Could you check a few things on this model? Use its own coordinates, in mm. Face numbers are marked on the shaded views. A direction names the side the tool comes from. Round coordinates to 2 decimals unless told otherwise and drop trailing zeros. Write each loop counter-clockwise with the first axis right and the second up, starting at its lowest first coordinate (ties: lowest second). Pieces come first, ordered by that corner, then holes. Notation, with made-up numbers: (36, 37) -> (92, 37) arc R15 cw to (92, 66) -> close; hole circle Ø5 at (49.5, 23). An arc over 180 degrees is marked (long way). Return JSON: item names as keys, results as strings.
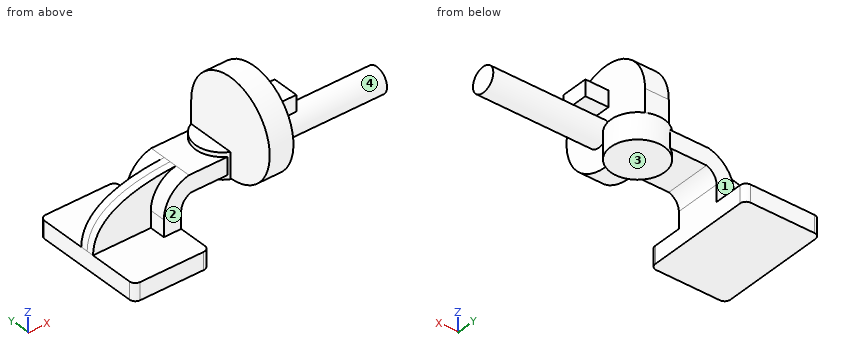
from build123d import *

# Parameters (mm, degrees)
F1_DEPTH  = 63.5
F0_W      = 21.3422756978
F0_H      = 19.05
F2_DEPTH  = 25.4
F3_DEPTH  = 7.9375
F5_R      = 6.35
F6_W      = 26.030293598
F6_H      = 52.8502463959
F7_DEPTH  = 25.4
F7_FACE_W = 26.030293598
F7_FACE_H = 52.8502463959
F9_W      = 29.2156040668
F9_H      = 17.6097750664
F10_DEPTH = 25.4
F12_R     = 13.6846052914
F13_DEPTH = 127


with BuildPart() as f1:
    # F0 (on Front) → F1 (new body, symmetric)
    with BuildSketch(Plane.XZ):
        Polygon((41.275, -9.525), (41.275, 9.525), (22.225, 9.525), (-41.275, 9.525), (-41.275, -9.525), align=None)
    extrude(amount=F1_DEPTH, both=True)

    # F0 (on Front) → F2 (join, symmetric)
    with BuildSketch(Plane.XZ):
        with BuildLine():
            Line((22.225, 9.525), (41.275, 9.525))
            Line((41.275, 9.525), (41.275, 27.7654680662))
            ThreePointArc((41.275, 27.7654680662), (44.31804227, 37.1119372292), (52.28054152, 42.8752))
            Line((52.28054152, 42.8752), (85.9294086695, 42.8752))
            Line((85.9294086695, 42.8752), (85.9294086695, 61.9252))
            Line((85.9294086695, 61.9252), (49.8789382336, 61.9252))
            ThreePointArc((49.8789382336, 61.9252), (30.0050422989, 49.7406107598), (22.225, 27.7654680662))
            Line((22.225, 27.7654680662), (22.225, 9.525))
        make_face()
        with Locations((96.6005465184, 52.4002)):
            Rectangle(F0_W, F0_H)
    extrude(amount=F2_DEPTH, both=True)

    # F0 (on Front) → F3 (join, symmetric)
    with BuildSketch(Plane.XZ):
        with BuildLine():
            Line((-41.275, 9.525), (22.225, 9.525))
            Line((22.225, 9.525), (22.225, 27.7654680662))
            ThreePointArc((22.225, 27.7654680662), (30.0050422989, 49.7406107598), (49.8789382336, 61.9252))
            add(Edge.make_bspline(
                [(-41.275, 9.525), (-40.6103878044, 51.4096161185), (12.72025149, 60.2582759139), (49.8789382336, 61.9252)],
                knots=[0, 0, 0, 0, 105.1419108421, 105.1419108421, 105.1419108421, 105.1419108421], degree=3))
        make_face()
    extrude(amount=F3_DEPTH, both=True)

    # F0 (on Front) → F4 (revolve)
    with BuildSketch(Plane.XZ):
        Polygon((107.2716843673, 61.9252), (107.2716843673, 42.8752), (107.2716843673, 38.1), (136.7294086695, 38.1), (136.7294086695, 66.675), (107.2716843673, 66.675), align=None)
    revolve(axis=Axis((107.2716843673, 0, 52.3875), (0, 0, -1)))

    # F5
    f5_edges = [f1.edges().sort_by_distance(p)[0] for p in [
        (41.275, -63.5, 0),
        (41.275, 63.5, 0),
        (-41.275, 63.5, 0),
        (-41.275, -63.5, 0),
    ]]
    fillet(f5_edges, radius=F5_R)

    # F6 (on face) → F7 (join)
    with BuildSketch(Plane.XY.offset(66.675)):
        with Locations((107.5195462284, -0.1220792231)):
            Rectangle(F6_W, F6_H)
    extrude(amount=F7_DEPTH)

    # F7_face (on face) → F8 (revolve)
    with BuildSketch(Plane(origin=(107.5195462284, -0.1220792231, 92.075), x_dir=(1, 0, 0), z_dir=(0, 0, 1))):
        Rectangle(F7_FACE_W, F7_FACE_H)
    revolve(axis=Axis((107.5195462284, -26.547202421, 92.075), (-1, 0, 0)))

    # F9 (on face) → F10 (join)
    with BuildSketch(Plane.YZ.offset(120.5346930274)):
        with Locations((-37.5394821167, 108.5370406508)):
            Rectangle(F9_W, F9_H)
    extrude(amount=F10_DEPTH)

    # F12 (on face) → F13 (join)
    with BuildSketch(Plane.YZ.offset(120.5346930274)):
        with Locations((-35.9719246626, 78.1719759107)):
            Circle(F12_R)
    extrude(amount=F13_DEPTH)


solid = f1.part
1) If I drill on probe 1 along Y at (x, z) = (2.5, 36); probe 2 along X at (y, z) = (-39.5, 4) (3 decimals); probe 3 along X at (y, z) = (-27.5, 124.5), over which ranges is the centre line in solid material (lowest first)? Write a range as [from, to].
Return value:
{"probe 1": "[-7.94, 7.94]", "probe 2": "[-41.275, 41.275]", "probe 3": "[94.5, 120.53]"}
2) I want a section at A-A, the plane z = 3.5. Please give me the cut outline in (x, y) (3 decimals), and give its area (3 significant figures).
Return value:
{"outline": "(-41.275, -57.15) arc R6.35 ccw to (-34.925, -63.5) -> (34.925, -63.5) arc R6.35 ccw to (41.275, -57.15) -> (41.275, 57.15) arc R6.35 ccw to (34.925, 63.5) -> (-34.925, 63.5) arc R6.35 ccw to (-41.275, 57.15) -> close", "area": "10,400 mm²"}
3) Will these pins go through, and if not, where does the flat tip stop? pin 1 Ø14 at (x, z) = (130.5, 111.5) entering from -Y; pin 2 Ø15.5 at (x, z) = (-6, 34.5) entering from +Y; pin 3 Ø4 at (y, z) = (-22.5, 108.5) entering from -X.
Return value:
{"pin 1": "y = -52.15", "pin 2": "y = 7.94", "pin 3": "x = 94.5"}
4) I want a section at D-D, the plane y = 21. Please give me the cut outline in (x, z) (3 decimals), and give its area (3 significant figures).
Return value:
{"outline": "(-41.275, -9.525) -> (41.275, -9.525) -> (41.275, 27.765) arc R15.875 cw to (52.281, 42.875) -> (86.614, 42.875) -> (86.614, 38.1) -> (127.93, 38.1) -> (127.93, 66.675) -> (120.535, 66.675) -> (120.535, 115.149) -> (94.504, 115.149) -> (94.504, 66.675) -> (86.614, 66.675) -> (86.614, 61.925) -> (49.879, 61.925) arc R34.925 ccw to (22.225, 27.765) -> (22.225, 9.525) -> (-41.275, 9.525) -> close", "area": "5,680 mm²"}
5) I want a section at C-C, the plane y = -18. Please give me the cut outline in (x, z) (3 decimals), and give its area (3 significant figures).
Return value:
{"outline": "(-41.275, -9.525) -> (41.275, -9.525) -> (41.275, 27.765) arc R15.875 cw to (52.281, 42.875) -> (83.953, 42.875) -> (83.953, 38.1) -> (130.59, 38.1) -> (130.59, 66.675) -> (120.535, 66.675) -> (120.535, 144.23) -> (94.504, 144.23) -> (94.504, 66.675) -> (83.953, 66.675) -> (83.953, 61.925) -> (49.879, 61.925) arc R34.925 ccw to (22.225, 27.765) -> (22.225, 9.525) -> (-41.275, 9.525) -> close", "area": "6,540 mm²"}
6) For the marked faces 1, 2, 3 and 4, which set-ups out of +Z, -Z, +X, -X, +Y, -Y let a thin tool reach every point of the face, with its end or its side?
Return value:
{"face 1": "+Z, -X, +Y", "face 2": "+Z, -X, -Y", "face 3": "-Z, +X, +Y, -Y", "face 4": "+X"}
7) I want a section at B-B, the plane y = -35. Please give me the cut outline in (x, z) (3 decimals).
Return value:
{"outline": "(-41.275, -9.525) -> (41.275, -9.525) -> (41.275, 9.525) -> (-41.275, 9.525) -> close; (94.504, 39.905) -> (120.535, 39.905) -> (120.535, 64.522) -> (247.535, 64.522) -> (247.535, 91.822) -> (120.535, 91.822) -> (120.535, 99.732) -> (145.935, 99.732) -> (145.935, 117.342) -> (120.535, 117.342) -> (120.535, 144.245) -> (94.504, 144.245) -> close"}
